The model under review builds one solid part; all positions refer to its coordinate system, in mm. A direction names the side the tool comes from. Coordinates: 2 decimals unless noted, no trailing zeros. Write each loop counter-clockwise with the first axis right and the second up, starting at its lowest first coordinate (ties: lowest second). Pieces come first, ordered by that corner, then holes.
1) Mouldability with a two-part tool opening along X and no side actions: class faces 1 (the flat face through (8.063, 12, 11)), 2 (the flat face through (-7, 13.5, 0)), 3 (the flat face through (2.59, 14.17, 0.18)), 4 (the flat face through (17.5, 5, 0)) as released by +X, released by -X, zero draft, split by the parting line, or undercut.
2) Add section A-A, the plane y = 9. State the section outline as (x, z) points.
3) Machinability: for faces 5 (the flat face through (-17.5, 5, 0)), 6 (the flat face through (16.063, 12, 8)), which of the approach directions +Z, -Z, +X, -X, +Y, -Y give a long, thin tool a straight path to every point of the face, cutting with its end or side? Answer none if there is none.
4) For P1, Ø8, axis at x = 1, z = -8.5, coming from the +Y side; P2, Ø0.6, axis at x = 7.5, y = 11, coming from the -Z side; P3, Ø1.5, axis at y = 13, z = 11, coming from the +X side, all flat-tipped, find the tip position at first contact; note any pin that passes through.
5) For line 1 (X direction, y = 10, z = 10); line 2 (Y direction, x = 9.5, z = 9.5); line 3 (Y direction, x = -2.5, z = 6), list the stretches that pass through material, from the lowest coordinate up.
from build123d import *

# Parameters (mm, degrees)
SKETCH1_W           = 35
SKETCH1_H           = 26
BOSS_EXTRUDE1_DEPTH = 10
SKETCH2_W           = 35
SKETCH2_H           = 26
BOSS_EXTRUDE3_DEPTH = 5
BOSS_EXTRUDE3_TAPER = 5
CUT_EXTRUDE1_DEPTH  = 35.745503475
CUT_EXTRUDE2_DEPTH  = 7
SKETCH5_W           = 12.5
SKETCH5_H           = 8.875113364
BOSS_EXTRUDE4_DEPTH = 3
BOSS_EXTRUDE4_TAPER = 4
SKETCH6_RX          = 4.540219564
SKETCH6_RY          = 3.227776247
BOSS_EXTRUDE5_DEPTH = 3
FILLET1_R           = 0.5
FILLET2_R           = 0.75


with BuildPart() as part:
    # Sketch1 → Boss-Extrude1 (new body)
    with BuildSketch(Plane(origin=(0, 0, 0), x_dir=(1, 0, 0), z_dir=(0, 1, 0))):
        Rectangle(SKETCH1_W, SKETCH1_H)
    extrude(amount=BOSS_EXTRUDE1_DEPTH)

    # Sketch2 → Boss-Extrude3 (add)
    with BuildSketch(Plane(origin=(0, 10, 0), x_dir=(1, 0, 0), z_dir=(0, 1, 0))):
        Rectangle(SKETCH2_W, SKETCH2_H)
    extrude(amount=BOSS_EXTRUDE3_DEPTH, taper=BOSS_EXTRUDE3_TAPER)

    # Sketch3 → Cut-Extrude1 (cut, through all)
    with BuildSketch(Plane.XY.offset(13)):
        Polygon((-17.500926093, 15), (3.562556682, 15), (1.806210322, 13.5), (-17.500926093, 13.5), align=None)
    extrude(amount=-CUT_EXTRUDE1_DEPTH, mode=Mode.SUBTRACT)

    # Sketch4 → Cut-Extrude2 (cut)
    with BuildSketch(Plane(origin=(0, 15, 0), x_dir=(1, 0, 0), z_dir=(0, 1, 0))):
        Polygon((8.062556682, -6.229226682), (8.062556682, -4.312556682), (7.312556682, -4.312556682), (7.312556682, -3.562556682), (8.062556682, -3.562556682), (16.062556682, -3.562556682), (16.062556682, -11.562556682), (8.062556682, -11.562556682), (8.062556682, -9.645896682), (7.312556682, -9.645896682), (7.312556682, -8.895896682), (8.062556682, -8.895896682), (8.062556682, -6.979226682), (7.312556682, -6.979226682), (7.312556682, -6.229226682), align=None)
    extrude(amount=-CUT_EXTRUDE2_DEPTH, mode=Mode.SUBTRACT)

    # Sketch5 → Boss-Extrude4 (add)
    with BuildSketch(Plane(origin=(0, 15, 0), x_dir=(1, 0, 0), z_dir=(0, 1, 0))):
        with Locations((10.562556682, 7.875)):
            Rectangle(SKETCH5_W, SKETCH5_H)
    extrude(amount=BOSS_EXTRUDE4_DEPTH, taper=BOSS_EXTRUDE4_TAPER)

    # Sketch6 → Boss-Extrude5 (add)
    with BuildSketch(Plane(origin=(0, 18, 0), x_dir=(1, 0, 0), z_dir=(0, 1, 0))):
        with Locations((10.562556682, 7.875)):
            Ellipse(SKETCH6_RX, SKETCH6_RY)
    extrude(amount=BOSS_EXTRUDE5_DEPTH)

    # Fillet1
    fillet1_edges = [part.edges().sort_by_distance(p)[0] for p in [
        (6.022337953, 21, -7.873042931),
    ]]
    fillet(fillet1_edges, radius=FILLET1_R)

    # Fillet2
    fillet2_edges = [part.edges().sort_by_distance(p)[0] for p in [
        (-7.693789678, 13.5, 12.693789678),
        (-7.693789678, 13.5, -12.693789678),
        (-17.193789678, 13.5, 0),
    ]]
    fillet(fillet2_edges, radius=FILLET2_R)


solid = part.part
Geometry results:
1. face 1: undercut
1. face 2: zero draft
1. face 3: released by -X
1. face 4: released by +X
2. outline: (-17.5, -13) - (17.5, -13) - (17.5, 13) - (-17.5, 13) - close; hole (7.31, 3.56) - (16.06, 3.56) - (16.06, 11.56) - (8.06, 11.56) - (8.06, 9.65) - (7.31, 9.65) - (7.31, 8.9) - (8.06, 8.9) - (8.06, 6.98) - (7.31, 6.98) - (7.31, 6.23) - (8.06, 6.23) - (8.06, 4.31) - (7.31, 4.31) - close
3. face 5: +Z, -Z, -X, +Y, -Y
3. face 6: +Y
4. P1: stops at y = 18
4. P2: stops at z = -12.94
4. P3: stops at x = 17.3
5. line 1: x = -17.5 to 8.06, 16.06 to 17.5
5. line 2: y = 0 to 8
5. line 3: y = 0 to 13.5
